```python
from build123d import *

# Parameters (mm, degrees)
SKETCH1_R           = 18.75
SKETCH1_W           = 80
SKETCH1_H           = 10
BOSS_EXTRUDE2_DEPTH = 4
CHAMFER2_SIZE2      = 4
CHAMFER2_SIZE       = 2
SKETCH1_3_R         = 1.375
BOSS_EXTRUDE3_DEPTH = 1
CHAMFER3_SIZE       = 0.5
CHAMFER4_SIZE       = 1
CHAMFER5_SIZE       = 2.5


# Some blends are built 0.0001 mm under size
with BuildPart() as part:
    # Sketch1 → Boss-Extrude2 (new body)
    # profile 1 of 2: a face of its own
    with BuildSketch(Plane(origin=(0, 0, 0), x_dir=(1, 0, 0), z_dir=(0, 1, 0))):
        Polygon((-25, 30), (-40, 30), (-40, -30), (40, -30), (40, 30), (25, 30), align=None)
        with BuildLine():
            ThreePointArc((-23.625, -25), (-25.972271824, -25.972271824), (-25, -23.625))
            ThreePointArc((-25, -23.625), (-24.027728176, -24.027728176), (-23.625, -25))
        make_face(mode=Mode.SUBTRACT)
        with BuildLine():
            ThreePointArc((-19.629554465, -12.920162208), (-21.542381919, -12.4375), (-21.003965926, -10.539611728))
            ThreePointArc((-21.003965926, -10.539611728), (-19.646750299, -10.569400091), (-18.976596989, -11.75))
            ThreePointArc((-18.976596989, -11.75), (-19.150881896, -12.420006168), (-19.629554465, -12.920162208))
        make_face(mode=Mode.SUBTRACT)
        with BuildLine():
            ThreePointArc((26.375, -25), (24.027728176, -25.972271824), (25, -23.625))
            ThreePointArc((25, -23.625), (25.972271824, -24.027728176), (26.375, -25))
        make_face(mode=Mode.SUBTRACT)
        with BuildLine():
            ThreePointArc((21.726596989, -11.75), (21.021603157, -12.950715093), (19.629554465, -12.920162208))
            ThreePointArc((19.629554465, -12.920162208), (19.681590821, -10.549284907), (21.726596989, -11.75))
        make_face(mode=Mode.SUBTRACT)
        with BuildLine():
            ThreePointArc((-25, 23.625), (-26.375, 25), (-25, 26.375))
            ThreePointArc((-25, 26.375), (-24.027728176, 25.972271824), (-23.625, 25))
            ThreePointArc((-23.625, 25), (-24.027728176, 24.027728176), (-25, 23.625))
        make_face(mode=Mode.SUBTRACT)
        with Locations(Location((0, 0, 0), (0, 0, 270))):
            Circle(SKETCH1_R, mode=Mode.SUBTRACT)
        with BuildLine():
            ThreePointArc((1.375, 23.5), (0.020115184, 22.125147143), (-1.374411461, 23.459773936))
            ThreePointArc((-1.374411461, 23.459773936), (-0.020115184, 24.874852857), (1.375, 23.5))
        make_face(mode=Mode.SUBTRACT)
        with BuildLine():
            ThreePointArc((25, 23.625), (23.625, 25), (25, 26.375))
            ThreePointArc((25, 26.375), (25.972271824, 25.972271824), (26.375, 25))
            ThreePointArc((26.375, 25), (25.972271824, 24.027728176), (25, 23.625))
        make_face(mode=Mode.SUBTRACT)
    # profile 2 of 2: a face of its own
    with BuildSketch(Plane(origin=(0, 0, 0), x_dir=(1, 0, 0), z_dir=(0, 1, 0))):
        with Locations((0, -35)):
            Rectangle(SKETCH1_W, SKETCH1_H)
    extrude(amount=BOSS_EXTRUDE2_DEPTH)

    # Chamfer2
    chamfer2_edges = [part.edges().sort_by_distance(p)[0] for p in [
        (0, 4, -18.75),
    ]]
    chamfer2_side = [part.faces().sort_by_distance(p)[0] for p in [
        (0, 4, -18.79),
    ]]
    chamfer(chamfer2_edges, length=CHAMFER2_SIZE - 0.0001, length2=CHAMFER2_SIZE2 - 0.0001, reference=chamfer2_side[0])  # a hair under: the kernel refuses the full size

    # Sketch1<3> → Boss-Extrude3 (add)
    with BuildSketch(Plane(origin=(0, 0, 0), x_dir=(1, 0, 0), z_dir=(0, 1, 0))):
        with Locations(Location((0, 23.5, 0), (0, 0, 270))):
            Circle(SKETCH1_3_R)
        with Locations(Location((20.351596989, -11.75, 0), (0, 0, 270))):
            Circle(SKETCH1_3_R)
        with Locations(Location((-20.351596989, -11.75, 0), (0, 0, 270))):
            Circle(SKETCH1_3_R)
    extrude(amount=BOSS_EXTRUDE3_DEPTH)

    # Chamfer3
    chamfer3_edges = [part.edges().sort_by_distance(p)[0] for p in [
        (-25, 0, 26.375),
        (-26.375, 0, -25),
        (23.625, 0, -25),
        (25, 0, 26.375),
    ]]
    chamfer(chamfer3_edges, length=CHAMFER3_SIZE)

    # Chamfer4
    chamfer4_edges = [part.edges().sort_by_distance(p)[0] for p in [
        (40, 2, 40),
        (-40, 2, 40),
    ]]
    chamfer(chamfer4_edges, length=CHAMFER4_SIZE)

    # Chamfer5
    # the kernel refuses this chamfer: 2.5 mm, written as the material it takes off along each edge
    with BuildSketch(Plane(origin=(40, 0, -36.42920747), x_dir=(0.0274958766105877, 0.9996219169112968, 0), z_dir=(0, 0, 1))) as chamfer5_piece_1:
        Polygon((CHAMFER5_SIZE * 0.999621916911, CHAMFER5_SIZE * 0.0274958766106), (-CHAMFER5_SIZE * 0.0274958766106, CHAMFER5_SIZE * 0.999621916911), (0, 0), align=None)
    extrude(amount=81.85841494, mode=Mode.SUBTRACT)
    with BuildSketch(Plane(origin=(-45.42920747, 0, 40), x_dir=(0, 0.9996219169112968, 0.0274958766105877), z_dir=(1, 0, 0))) as chamfer5_piece_2:
        Polygon((CHAMFER5_SIZE * 0.999621916911, -CHAMFER5_SIZE * 0.0274958766106), (-CHAMFER5_SIZE * 0.0274958766106, -CHAMFER5_SIZE * 0.999621916911), (0, 0), align=None)
    extrude(amount=90.85841494, mode=Mode.SUBTRACT)
    with BuildSketch(Plane(origin=(-40, 0, -36.42920747), x_dir=(-0.0274958766105877, 0.9996219169112968, 0), z_dir=(0, 0, 1))) as chamfer5_piece_3:
        Polygon((CHAMFER5_SIZE * 0.999621916911, -CHAMFER5_SIZE * 0.0274958766106), (-CHAMFER5_SIZE * 0.0274958766106, -CHAMFER5_SIZE * 0.999621916911), (0, 0), align=None)
    extrude(amount=81.85841494, mode=Mode.SUBTRACT)


solid = part.part
```
Here's how the part is built. I have some questions about the finished solid (model axes, mm). A direction names the side the tool comes from. Coordinates: 2 decimals unless noted, no trailing zeros. Order: outer loops, then holes, each group sorted by start corner. A loop starts at its lowest first (then second) coordinate and runs counter-clockwise, first axis right, second up.
Item 1: Thinking about a two-plate mould opening in X: for faces 3 (the face through (-38.8, 1.3, 4.3)), 4 (the face through (-20, 1, 12)), 5 (the face through (-0.6, 1.3, 38.8)), 6 (the face through (38.8, 1.3, 4.3)), which applies, pulls with the +X half, pulls with the -X half, needs draft (parallel to the pull), parting line crosses it, or undercut?
Response values:
face 3: pulls with the -X half
face 4: undercut
face 5: needs draft
face 6: pulls with the +X half
Item 2: Which directions (+Z, -Z, +X, -X, +Y, -Y) give clear straight access to the entire face, cutting with the end or side of a thin tool? Please do faces 1 (the face through (9, 0, 18)), 2 (the face through (0, 1, -24)).
Response values:
face 1: +Z, -Z, +X, -X, -Y
face 2: +Y
Item 3: I need wall thicknesses on probe 1 along X at (y, z) = (1.5, 25) (3 decimals); probe 2 along X at (y, z) = (2.55, 25) (3 decimals); probe 3 along Z at (x, y) = (-25, 3) (3 decimals). Which ranges of each line are inside material? Lowest first, please.
Response values:
probe 1: x = -39 to -26.375, -23.625 to 23.625, 26.375 to 39
probe 2: x = -40 to -26.375, -23.625 to 23.625, 26.375 to 40
probe 3: z = -30 to -26.375, -23.625 to 23.625, 26.375 to 40
Item 4: If we section it at B-B, the plane z = 31: List the corners of the cut face in (x, y) for me.
Response values:
outline: (-40, 2.5) - (-37.5, 0) - (37.5, 0) - (40, 2.5) - (40, 4) - (-40, 4) - close
Item 5: I'm going to push a flat-ended pin straight in: pin 1 Ø3 at (x, z) = (-25, 25) entering from -Y (3 decimals). Where does the tip first touch, or does it pass through?
Response values:
pin 1: stops at y = 0.375
